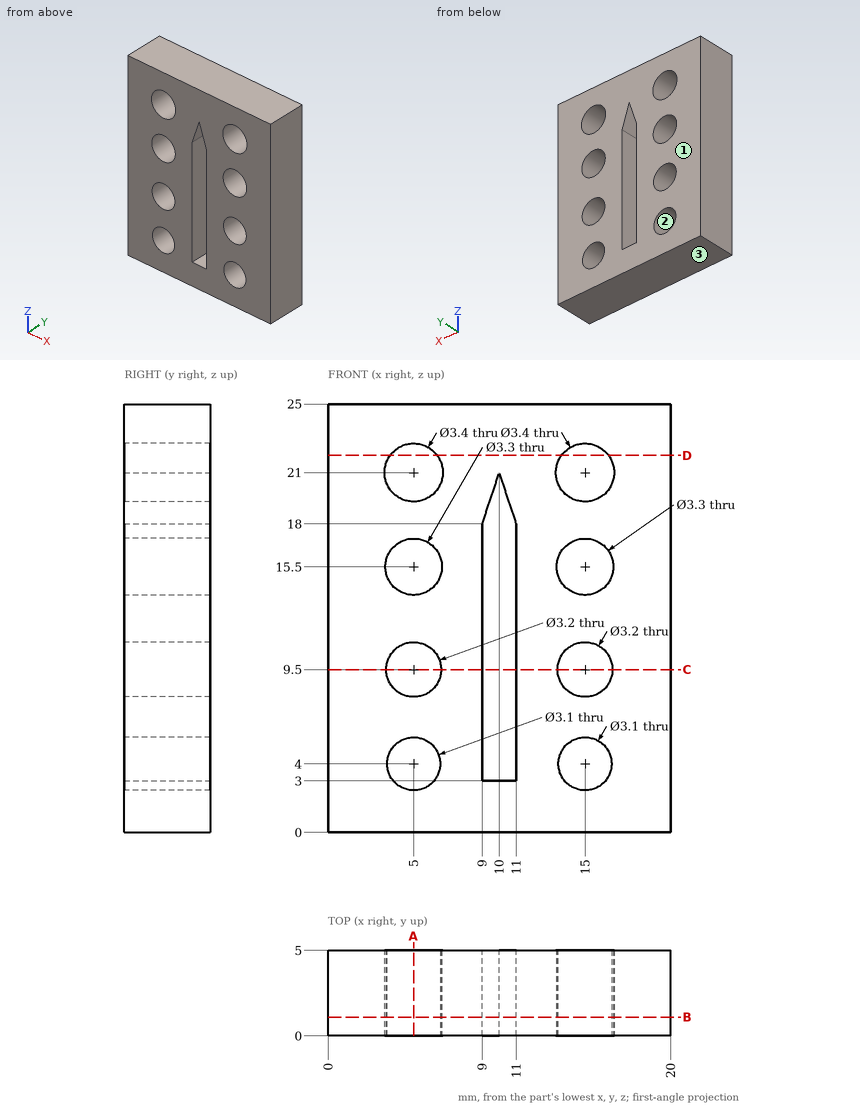
The drawing under review shows one solid part. Ordinate dimensions are in mm from its lowest x, y, z. Round coordinates to 2 decimals unless told otherwise and drop trailing zeros. Write each loop counter-clockwise with the first axis right and the second up, starting at its lowest first coordinate (ties: lowest second). Pieces come first, ordered by that corner, then holes. Notation, with made-up numbers: (68, 6.25) - (103, 6.25) arc R15 cw to (103, 15.25) - close; hole circle Ø4 at (83, 52.5). An arc over 180 degrees is marked (long way). One line per question, with ' | ' between items.
Item 1: Add section D-D, the plane z = 22. Give the boundary of the cut face in (x, y), then the cut area to 3 significant figures.
Resolved:
outline: (0, 0) - (3.63, 0) - (3.63, 5) - (0, 5) - close; (6.37, 0) - (13.63, 0) - (13.63, 5) - (6.37, 5) - close; (16.37, 0) - (20, 0) - (20, 5) - (16.37, 5) - close | area: 72.5 mm2
Item 2: The part is to be moulded in two halves that separate along Z. For the marked faces 1, 2 and 3, say which applies: pulls with the +Z half, pulls with the -Z half, needs draft (parallel to the pull), parting line crosses it, or undercut.
Resolved:
face 1: needs draft | face 2: undercut | face 3: pulls with the -Z half
Item 3: Add section A-A, the plane x = 5. Give the boundary of the cut face in (y, z), then the cut area to 3 significant figures.
Resolved:
outline: (0, 0) - (5, 0) - (5, 2.45) - (0, 2.45) - close; (0, 5.55) - (5, 5.55) - (5, 7.9) - (0, 7.9) - close; (0, 11.1) - (5, 11.1) - (5, 13.85) - (0, 13.85) - close; (0, 17.15) - (5, 17.15) - (5, 19.3) - (0, 19.3) - close; (0, 22.7) - (5, 22.7) - (5, 25) - (0, 25) - close | area: 60.0 mm2
Item 4: To check wall thickness, follow probe 1 along Z at (x, y) = (15, 1.2); probe 2 along X at (y, z) = (4.55, 5.75); probe 3 along X at (y, z) = (4.6, 22.5). State the ranges of each line that lie inside material, in increasing order.
Resolved:
probe 1: z = 0 to 2.45, 5.55 to 7.9, 11.1 to 13.85, 17.15 to 19.3, 22.7 to 25 | probe 2: x = 0 to 9, 11 to 20 | probe 3: x = 0 to 4.2, 5.8 to 14.2, 15.8 to 20
Item 5: Add section C-C, the plane z = 9.5. Give the boundary of the cut face in (x, y), then the cut area to 3 significant figures.
Resolved:
outline: (0, 0) - (3.4, 0) - (3.4, 5) - (0, 5) - close; (6.6, 0) - (9, 0) - (9, 5) - (6.6, 5) - close; (11, 0) - (13.4, 0) - (13.4, 5) - (11, 5) - close; (16.6, 0) - (20, 0) - (20, 5) - (16.6, 5) - close | area: 58.0 mm2
Item 6: Add section B-B, the plane y = 1.1. State how many separate pieces and enclosed holes the cut face has, then the cut area to 3 significant figures.
Resolved:
separate pieces: 1 | enclosed holes: 9 | area: 401 mm2
Item 7: For P1, Ø3, axis at x = 15, z = 15.5, coming from the -Y side, flat-tipped, find the tip position at first contact; note if it passes through.
Resolved:
P1: passes through
